from build123d import *

# Parameters (mm, degrees)
SKETCH_1_W      = 35
SKETCH_1_H      = 35
EXTRUDE_1_DEPTH = 25
CHAMFER_1_SIZE  = 5
SKETCH_2_R      = 11
EXTRUDE_2_DEPTH = 2
SKETCH_3_R      = 8.5
EXTRUDE_3_DEPTH = 11


with BuildPart() as part:
    # Эскиз1 → Бобышка-Вытянуть1 (new body)
    with BuildSketch(Plane.XY):
        Rectangle(SKETCH_1_W, SKETCH_1_H)
    extrude(amount=EXTRUDE_1_DEPTH)

    # Фаска1
    chamfer_1_edges = [part.edges().sort_by_distance(p)[0] for p in [
        (17.5, -17.5, 12.5),
        (-17.5, -17.5, 12.5),
        (-17.5, 17.5, 12.5),
        (17.5, 17.5, 12.5),
    ]]
    chamfer(chamfer_1_edges, length=CHAMFER_1_SIZE)

    # Эскиз2 → Бобышка-Вытянуть2 (add)
    with BuildSketch(Plane(origin=(0, 0, 0), x_dir=(-1, 0, 0), z_dir=(0, 0, -1))):
        Circle(SKETCH_2_R)
    extrude(amount=EXTRUDE_2_DEPTH)

    # Эскиз3 → Бобышка-Вытянуть3 (add)
    with BuildSketch(Plane(origin=(0, 0, -2), x_dir=(-1, 0, 0), z_dir=(0, 0, -1))):
        Circle(SKETCH_3_R)
    extrude(amount=EXTRUDE_3_DEPTH)


solid = part.part
The listing builds one solid part. Answer for the finished solid, in the listing's coordinates (mm). A direction names the side the tool comes from. Round coordinates to 2 decimals unless told otherwise and drop trailing zeros. Order: outer loops, then holes, each group sorted by start corner. A loop starts at its lowest first (then second) coordinate and runs counter-clockwise, first axis right, second up. Notation, with made-up numbers: (18.25, 86.5) -> (62.25, 86.5) arc R20 cw to (62.25, 111.5) -> close; hole circle Ø6 at (-30.75, 51.5). An arc over 180 degrees is marked (long way). One line per item, written item: value.
Item 1: Find section A-A, the plane z = 21. Give the vertices of the cut face in (x, y).
Taken from the geometry:
outline: (-17.5, -12.5) -> (-12.5, -17.5) -> (12.5, -17.5) -> (17.5, -12.5) -> (17.5, 12.5) -> (12.5, 17.5) -> (-12.5, 17.5) -> (-17.5, 12.5) -> close
Item 2: For faces 1 (the flat face through (0, 0, -13)), 2 (the flat face through (-3.2, -8.1, -2)), determine the directions among +Z, -Z, +X, -X, +Y, -Y from which every point of the face is accessible in a straight line to the end or side of a thin tool.
Taken from the geometry:
face 1: -Z, +X, -X, +Y, -Y
face 2: -Z
Item 3: Given P1, Ø3, axis at y = -1.5, z = -8.5, coming from the -X side, flat-ended and moving along its own axis, determine where the tip first touches the part or whether it passes through.
Taken from the geometry:
P1: stops at x = -8.5
Item 4: Find section B-B, the plane x = 0. Give the vertices of the cut face in (y, z).
Taken from the geometry:
outline: (-17.5, 0) -> (-11, 0) -> (-11, -2) -> (-8.5, -2) -> (-8.5, -13) -> (8.5, -13) -> (8.5, -2) -> (11, -2) -> (11, 0) -> (17.5, 0) -> (17.5, 25) -> (-17.5, 25) -> close
Item 5: Find section D-D, the plane x = 12. Give the vertices of the cut face in (y, z).
Taken from the geometry:
outline: (-17.5, 0) -> (17.5, 0) -> (17.5, 25) -> (-17.5, 25) -> close
Item 6: Straight lines are drawn through the part: L1, parallel to Z at x = -5.5, y = 14.5; L2, parallel to Z at x = 1.5, y = 8.5; L3, parallel to Y at x = -13, z = 13. For each, find the intervals that lie inside material, in ascending order.
Taken from the geometry:
L1: z = 0 to 25
L2: z = -2 to 25
L3: y = -17 to 17
